from build123d import *

# Parameters (mm, degrees)
BASEHEAD_DEPTH     = 3.65
INDENT_START       = -0.45625
INDENT_2_OUTLINE_R = 3.5
INDENT_2_DEPTH     = 0.45625
SKETCH4_W          = 0.5
SKETCH4_H          = 10.618802154


# Read off the part's stored shape, not the designer's step: Indent
with BuildPart() as part:
    # Sketch1 → BaseHead (new body)
    with BuildSketch(Plane(origin=(0, 0, 0), x_dir=(0, 0, -1), z_dir=(1, 0, 0))):
        Polygon((4, 2.309401077), (4, -2.309401077), (0, -4.618802154), (-4, -2.309401077), (-4, 2.309401077), (0, 4.618802154), align=None)
    extrude(amount=BASEHEAD_DEPTH)

    # Indent outline → Indent (revolve)
    with BuildSketch(Plane.YX):
        Polygon((2.5, 3.65), (2.5, 13.205), (2.055, 13.65), (0, 13.65), (0, 3.65), align=None)
    revolve(axis=Axis((0, 0, 0), (1, 0, 0)))

    # Indent 2 outline → Indent 2 (cut)
    with BuildSketch(Plane.ZY.offset(INDENT_START)):
        with Locations((0.033212245, 0.192376607)):
            Circle(INDENT_2_OUTLINE_R)
    extrude(amount=INDENT_2_DEPTH, mode=Mode.SUBTRACT)

    # Sketch3 → HeadChamfer (revolve, cut)
    with BuildSketch(Plane.XY, mode=Mode.PRIVATE) as headchamfer_sk:
        Polygon((0, 4), (3.244016936, 9.618802154), (3.244016936, 14.618802154), (-10, 14.618802154), (-10, 4), align=None)
    revolve(headchamfer_sk.sketch.rotate(Axis((0, 0, 0), (1, 0, 0)), 90), axis=Axis((0, 0, 0), (1, 0, 0)), mode=Mode.SUBTRACT)

    # Sketch4 → BearingFace (revolve, cut)
    with BuildSketch(Plane.XY, mode=Mode.PRIVATE) as bearingface_sk:
        with Locations((3.4, 9.309401077)):
            Rectangle(SKETCH4_W, SKETCH4_H)
    revolve(bearingface_sk.sketch.rotate(Axis((0, 0, 0), (1, 0, 0)), 90), axis=Axis((0, 0, 0), (1, 0, 0)), mode=Mode.SUBTRACT)


solid = part.part
Source: CAD feature listing. Evaluate the final solid. Frame: model axes, mm. A direction names the side the tool comes from. Give positions to 0.01 mm unless a question says otherwise; leave off trailing zeros. Write each loop counter-clockwise with the first axis right and the second up, starting at its lowest first coordinate (ties: lowest second). Pieces come first, ordered by that corner, then holes. Notation, with made-up numbers: M -32.75,68 L 10.25,68 A23 cw 10.25,97 Z; hole C 62,34 d2. An arc over 180 degrees is marked long. Return JSON: item names as keys, results as strings. Group by question number.
1) Set-up query: faces 1 (the face through (3.15, -2.1, -3.6)), 2 (the face through (0.456, 0, 0)), 3 (the face through (8.49, -0.54, -2.44)). Return all of +Z, -Z, +X, -X, +Y, -Y with unobstructed straight access to the full face (end or side cutting, diameter ignored); none if empty.
2) Cut plane A-A, the plane x = 11.75. Output: boundary loops of the cut face in (y, z).
3) Material intervals for line 1 along X through (y, z) = (-0.5, -1.25); line 2 along X through (y, z) = (-3, 0.5); line 3 along Y through (x, z) = (8.25, 1.5), sorted ascending. Write a range as [from, to].
4) Pull-direction query (Z, two-part tool) for faces 4 (the face through (0.087, 2.084, 3.589)), 5 (the face through (0.087, -2.084, -3.589)), 6 (the face through (0.231, 3.663, -0.422)), 7 (the face through (3.15, -2.1, 3.6)); classes: pulls with the +Z half, pulls with the -Z half, needs draft (parallel to the pull), parting line crosses it, or undercut.
5) Pin query (flat end, axial travel): P1, Ø3, axis at x = 5.5, z = -1.5, coming from the +Y side; P2, Ø2, axis at y = -2, z = 3.5, coming from the +X side; P3, Ø1, axis at y = -2.5, z = 1, coming from the +X side. Return the tip coordinate at first contact, or that it passes through.
Recorded:
{
 "1": {"face 1": "-Z, +X, -Y", "face 2": "-X", "face 3": "+X"},
 "2": {"outline": "C 0,0 d5"},
 "3": {"line 1": "x = [0.46, 13.65]", "line 2": "x = [0.46, 3.65]", "line 3": "y = [-2, 2]"},
 "4": {"face 4": "pulls with the +Z half", "face 5": "pulls with the -Z half", "face 6": "undercut", "face 7": "needs draft"},
 "5": {"P1": "stops at y = 2.5", "P2": "stops at x = 3.65", "P3": "stops at x = 13.51"}
}
